For this review, take the finished solid that the model builds, in its own axes (mm). Face numbers are marked on the shaded views. A direction names the side the tool comes from. Round coordinates to 2 decimals unless told otherwise and drop trailing zeros. Order: outer loops, then holes, each group sorted by start corner. A loop starts at its lowest first (then second) coordinate and runs counter-clockwise, first axis right, second up. Notation, with made-up numbers: (46, -4) - (77, -4) arc R8 ccw to (77, 1) - close; hole circle Ø10 at (22.5, -19.5). An arc over 180 degrees is marked (long way). One line per item, written item: value.
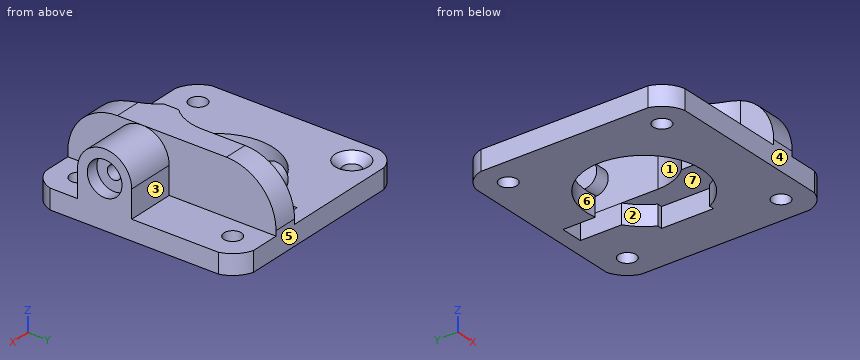
```python
from build123d import *

# Parameters (mm, degrees)
CROQUIS2_R                                           = 1.75875
SALIENTE_EXTRUIR1_DEPTH                              = 4
CROQUIS3_W                                           = 4.82
CROQUIS3_H                                           = 42
SALIENTE_EXTRUIR2_DEPTH                              = 11
CROQUIS5_R                                           = 2.515
SALIENTE_EXTRUIR3_DEPTH                              = 3
CROQUIS6_W                                           = 2.7
CROQUIS6_H                                           = 3
SALIENTE_EXTRUIR4_DEPTH                              = 11
REDONDEO1_R                                          = 10
CORTAR_EXTRUIR1_REACH                                = 37.805
CROQUIS8_R                                           = 1.4
REDONDEO2_R                                          = 10
CROQUIS9_R                                           = 1.4
SALIENTE_EXTRUIR5_DEPTH                              = 9.75
CROQUIS10_R                                          = 3.5
CORTAR_EXTRUIR2_DEPTH                                = 2.5
REFRENTADO_PARA_TORNILLO_TAP_N_CON_CABEZ_D           = 3.3
REFRENTADO_PARA_TORNILLO_TAP_N_CON_CABEZ_CSINK_D     = 6.72
REFRENTADO_PARA_TORNILLO_TAP_N_CON_CABEZ_CSINK_ANGLE = 90


with BuildPart() as part:
    # Croquis2 → Saliente-Extruir1 (new body)
    with BuildSketch(Plane.XY):
        with BuildLine():
            Line((-10.901498769, 16.692640248), (-10.901498769, -17.009890921))
            ThreePointArc((-10.901498769, -17.009890921), (-9.344660807, -19.660096087), (-6.631805383, -21.105))
            Line((-6.631805383, -21.105), (27.102123863, -21.105))
            ThreePointArc((27.102123863, -21.105), (29.626712806, -19.633211575), (31.098501231, -17.108622633))
            Line((31.098501231, -17.108622633), (31.098501231, 16.847284537))
            ThreePointArc((31.098501231, 16.847284537), (29.679453987, 19.385312533), (27.194272919, 20.895))
            Line((27.194272919, 20.895), (-6.699139018, 20.895))
            ThreePointArc((-6.699139018, 20.895), (-9.401498769, 19.395), (-10.901498769, 16.692640248))
        make_face()
        with Locations((-5.428998769, 15.4225)):
            Circle(CROQUIS2_R, mode=Mode.SUBTRACT)
        with Locations((25.571001231, 15.4225)):
            Circle(CROQUIS2_R, mode=Mode.SUBTRACT)
        with Locations((25.571001231, -15.5775)):
            Circle(CROQUIS2_R, mode=Mode.SUBTRACT)
        with Locations((-5.428998769, -15.5775)):
            Circle(CROQUIS2_R, mode=Mode.SUBTRACT)
        with BuildLine():
            Line((20.363327993, -5.226), (21.350001231, -5.226))
            Line((21.350001231, -5.226), (21.350001231, 5.225999923))
            Line((21.350001231, 5.225999923), (20.363328032, 5.225999923))
            ThreePointArc((20.363328032, 5.225999923), (18.722008699, 7.645662593), (16.526001231, 9.57601173))
            Line((16.526001231, 9.57601173), (16.526001231, 17.886))
            Line((16.526001231, 17.886), (12.011001231, 17.886))
            Line((12.011001231, 17.886), (12.011001231, 11.390753987))
            ThreePointArc((12.011001231, 11.390753987), (-0.271544795, -5.190509466), (20.363327993, -5.226))
        make_face(mode=Mode.SUBTRACT)
    extrude(amount=SALIENTE_EXTRUIR1_DEPTH)

    # Croquis3 → Saliente-Extruir2 (add)
    with BuildSketch(Plane.XY.offset(4)):
        with Locations((18.938501231, -0.105)):
            Rectangle(CROQUIS3_W, CROQUIS3_H)
    extrude(amount=SALIENTE_EXTRUIR2_DEPTH)

    # Croquis5 → Saliente-Extruir3 (add)
    with BuildSketch(Plane.ZY.offset(-16.528501231)):
        with Locations(Location((9.53, 14.775, 0), (0, 0, 90))):
            Circle(CROQUIS5_R)
    extrude(amount=SALIENTE_EXTRUIR3_DEPTH)

    # Croquis6 → Saliente-Extruir4 (add)
    with BuildSketch(Plane.XY.offset(15)):
        with Locations((15.178501231, -6.105)):
            Rectangle(CROQUIS6_W, CROQUIS6_H)
    extrude(amount=-SALIENTE_EXTRUIR4_DEPTH)

    # Redondeo1
    # the kernel refuses this fillet: 10 mm, written as the material it adds along each edge
    with BuildSketch(Plane(origin=(16.528501231, -4.605, 15), x_dir=(0, 1, 0), z_dir=(0, 0, -1))) as redondeo1_piece_1:
        with BuildLine():
            CenterArc((6.83447145, -10), REDONDEO1_R, 90, 43.113605946)
            Line((0, -2.7), (-0.136689429, -2.554))
            ThreePointArc((-0.136689429, -2.554), (-0.2, -1.35), (-0.2, 0))
            Line((-0.2, 0), (0, 0.2))
            Line((0, 0.2), (6.83447145, 0.2))
            Line((6.83447145, 0.2), (6.83447145, 0))
        make_face()
    extrude(amount=11)
    with BuildSketch(Plane(origin=(16.528501231, -7.605, 15), x_dir=(0, -1, 0), z_dir=(0, 0, -1))) as redondeo1_piece_2:
        with BuildLine():
            CenterArc((6.83447145, 10), REDONDEO1_R, 226.886394054, 43.113605946)
            Line((0, 2.7), (-0.136689429, 2.554))
            ThreePointArc((-0.136689429, 2.554), (-0.2, 1.35), (-0.2, 0))
            Line((-0.2, 0), (0, -0.2))
            Line((0, -0.2), (6.83447145, -0.2))
            Line((6.83447145, -0.2), (6.83447145, 0))
        make_face()
    extrude(amount=11)

    # Croquis8 → Cortar-Extruir1 (cut, up to next)
    with BuildSketch(Plane.ZY.offset(-13.828501231), mode=Mode.PRIVATE) as cortar_extruir1_sk1:
        with Locations((9.53, -6.125)):
            Circle(CROQUIS8_R)
    cortar_extruir1_tool1 = extrude(cortar_extruir1_sk1.sketch, amount=-CORTAR_EXTRUIR1_REACH, mode=Mode.PRIVATE) & part.part
    add(cortar_extruir1_tool1.solids().sort_by_distance((13.828501, -6.125, 9.53))[0], mode=Mode.SUBTRACT)

    # Redondeo2
    redondeo2_edges = [part.edges().sort_by_distance(p)[0] for p in [
        (18.938501231, -21.105, 15),
        (18.938501231, 20.895, 15),
    ]]
    fillet(redondeo2_edges, radius=REDONDEO2_R)

    # Croquis9 → Saliente-Extruir5 (add)
    with BuildSketch(Plane(origin=(21.348501231, 0, 0), x_dir=(0, 0, -1), z_dir=(1, 0, 0))):
        with BuildLine():
            Line((-9.53, -0.655), (-4, -0.655))
            Line((-4, -0.655), (-4, -11.595))
            Line((-4, -11.595), (-9.53, -11.595))
            ThreePointArc((-9.53, -11.595), (-15, -6.125), (-9.53, -0.655))
        make_face()
        with Locations(Location((-9.53, -6.125, 0), (0, 0, 180))):
            Circle(CROQUIS9_R, mode=Mode.SUBTRACT)
    extrude(amount=SALIENTE_EXTRUIR5_DEPTH)

    # Croquis10 → Cortar-Extruir2 (cut)
    with BuildSketch(Plane(origin=(31.098501231, 0, 0), x_dir=(0, 0, -1), z_dir=(1, 0, 0))):
        with Locations(Location((-9.53, -6.125, 0), (0, 0, 90))):
            Circle(CROQUIS10_R)
    extrude(amount=-CORTAR_EXTRUIR2_DEPTH, mode=Mode.SUBTRACT)

    # Refrentado para tornillo tapón con cabeza plana de clavija de M31 (through all)
    with Locations(Plane.XY.offset(4)):
        with Locations((-5.428998769, 15.4225)):
            CounterSinkHole(REFRENTADO_PARA_TORNILLO_TAP_N_CON_CABEZ_D / 2, REFRENTADO_PARA_TORNILLO_TAP_N_CON_CABEZ_CSINK_D / 2, counter_sink_angle=REFRENTADO_PARA_TORNILLO_TAP_N_CON_CABEZ_CSINK_ANGLE)


solid = part.part
```
Item 1: The part is to be moulded in two halves that separate along Y. For the marked faces 4, 5, 6 and 7, say which applies: +Y half, -Y half, draft (parallel to the pull), parting line (faces both ways), or undercut.
Returned:
face 4: -Y half
face 5: +Y half
face 6: undercut
face 7: undercut
Item 2: Machinability: for the marked faces 1, 2 and 3, which of the approach directions +Z, -Z, +X, -X, +Y, -Y give a long, thin tool a straight path to every point of the face, cutting with its end or side? Answer none if there is none.
Returned:
face 1: +Z, -Z, -X
face 2: -Z
face 3: +Z, +X, +Y
Item 3: For P1, Ø4.5, axis at x = -5.43, y = -15.58, coming from the +Z side; P2, Ø6, axis at y = 6, z = 9.5, coming from the -X side; P3, Ø8, axis at y = 12.5, z = 12.5, coming from the -X side; P4, Ø4.5, axis at x = 25.57, y = 15.42, coming from the -Z side, all flat-tipped, find the tip position at first contact; note any pin that passes through.
Returned:
P1: z = 4
P2: x = 16.53
P3: x = 13.53
P4: z = 0
Item 4: Take a section at B-B (x = 9). Write out the cut boundary in (y, z) (3 decimals).
Returned:
outline: (-21.105, 0) - (-11.509, 0) - (-11.509, 4) - (-21.105, 4) - close; (11.509, 0) - (20.895, 0) - (20.895, 4) - (11.509, 4) - close
Item 5: Take a section at D-D (y = 16). Count the separate pieces of the cut face and the enclosed holes in it, plus the area to 3 significant figures.
Returned:
separate pieces: 4
enclosed holes: 0
area: 180 mm^2
Item 6: Wall thickness on line 1 (Y direction, x = 27, z = 0.5) (3 decimals); line 2 (X direction, y = 15.5, z = 3.25); line 3 (Z direction, x = -3, y = -12.5): over which ranges is each line inside the solid? List them lowest first.
Returned:
line 1: -21.105 to -16.603, -14.552 to 14.397, 16.448 to 20.895
line 2: -10.9 to -8.04, -2.82 to 12.01, 16.53 to 23.81, 27.33 to 31.1
line 3: 0 to 4
Item 7: Take a section at A-A (y = 4). Write out the cut boundary in (x, z), plus the area to 3 significant figures.
Returned:
outline: (-10.9, 0) - (-0.79, 0) - (-0.79, 4) - (-10.9, 4) - close; (16.53, 4) - (21.35, 4) - (21.35, 15) - (16.53, 15) - close; (21.35, 0) - (31.1, 0) - (31.1, 4) - (21.35, 4) - close
area: 132 mm^2
Item 8: Take a section at C-C (z = 4.5). Write out the cut boundary in (x, y) (1 decimal).
Returned:
outline: (13.8, -7.6) arc R10 cw to (16.5, -14.4) - (16.5, -21.1) - (21.3, -21.1) - (21.3, -11.6) - (31.1, -11.6) - (31.1, -0.7) - (21.3, -0.7) - (21.3, 20.9) - (16.5, 20.9) - (16.5, 2.2) arc R10 cw to (13.8, -4.6) - close
